from build123d import *

# Parameters (mm, degrees)
SKETCH_2_R          = 20
EXTRUDE_2_DEPTH     = 50
SKETCH_3_R          = 10
SKETCH_3_W          = 50
SKETCH_3_H          = 8
EXTRUDE_3_DEPTH     = 30
EXTRUDE_START       = -12
SKETCH_4_R          = 10
EXTRUDE_4_DEPTH     = 12
SKETCH_5_R          = 13
SKETCH_5_R_2        = 5.5
CUT_EXTRUDE_1_DEPTH = 89.593995864


with BuildPart() as part:
    # Эскиз2 → Бобышка-Вытянуть2 (new body)
    with BuildSketch(Plane.XY):
        Circle(SKETCH_2_R)
    extrude(amount=EXTRUDE_2_DEPTH)

    # Эскиз3 → Бобышка-Вытянуть3 (add)
    with BuildSketch(Plane.XY.offset(50)):
        with Locations((-50, 0)):
            Circle(SKETCH_3_R)
        with Locations((-25, 0)):
            Rectangle(SKETCH_3_W, SKETCH_3_H)
    extrude(amount=-EXTRUDE_3_DEPTH)

    # Эскиз4 → Бобышка-Вытянуть4 (add)
    with BuildSketch(Plane.XY.offset(50).offset(EXTRUDE_START)):
        with BuildLine():
            Line((-10.645829468, -16.931223079), (26.496890419, -40.285416693))
            ThreePointArc((26.496890419, -40.285416693), (24.748737342, -24.748737342), (40.285416693, -26.496890419))
            Line((40.285416693, -26.496890419), (16.931223079, 10.645829468))
            ThreePointArc((16.931223079, 10.645829468), (14.142135624, -14.142135624), (-10.645829468, -16.931223079))
        make_face()
        with Locations((31.819805153, -31.819805153)):
            Circle(SKETCH_4_R)
    extrude(amount=EXTRUDE_4_DEPTH)

    # Эскиз5 → Вырез-Вытянуть1 (cut, through all)
    with BuildSketch(Plane.XY.offset(50)):
        Circle(SKETCH_5_R)
        with Locations((-50, 0)):
            Circle(SKETCH_5_R_2)
        with Locations((31.819805153, -31.819805153)):
            Circle(SKETCH_5_R_2)
    extrude(amount=-CUT_EXTRUDE_1_DEPTH, mode=Mode.SUBTRACT)


solid = part.part
Could you check a few things on this model? Use its own coordinates, in mm. A direction names the side the tool comes from. Coordinates: 2 decimals unless noted, no trailing zeros. Write each loop counter-clockwise with the first axis right and the second up, starting at its lowest first coordinate (ties: lowest second). Pieces come first, ordered by that corner, then holes. Notation, with made-up numbers: (26.25, -28.5) - (35.25, -28.5) arc R12 ccw to (35.25, -5.5) - close; hole circle Ø2 at (33.5, -23.5). An arc over 180 degrees is marked (long way). Put each result on its own line as item: value. Start each with the question number.
Q1. I want a section at D-D on y = 0. Write out the boundary of the cut face in (x, z) (3 decimals).
Q2. I want a section at B-B on y = -28. Write out the boundary of the cut face in (x, z).
Q3. Thinking about a two-plate mould opening in X: for faces 4 (the cylindrical face through (-55.495, 0.242, 35.21)), 5 (the flat face through (28.772, -8.186, 43.916)), 6 (the cylindrical face through (-60, 0, 35)), 7 (the flat face through (-40, 0, 20)), which applies, pulls with the +X half, pulls with the -X half, needs draft (parallel to the pull), parting line crosses it, or undercut?
Q4. I want a section at C-C on z = 21.5. Write out the boundary of the cut face in (x, y).
Q5. Which directions (+Z, -Z, +X, -X, +Y, -Y) give clear straight access to the entire face, cutting with the end or side of a thin tool? Please do faces 1 (the flat face through (-30, 4, 35)), 2 (the cylindrical face through (-2.6, 19.83, 19.09)), 3 (the flat face through (-30, -4, 35)).
Q6. Please list where these lines run through material, in increasing order: L1, parallel to X at y = -6, z = 43.5; L2, parallel to Y at x = -33, z = 25; L3, parallel to X at y = -7.5, z = 28.
Q7. I'm going to push flat-ended pins straight in: P1, Ø6.5, axis at x = -32.5, z = 29.5, coming from the -Y side; P2, Ø14.5, axis at x = -50, y = 0, coming from the -Z side; P3, Ø6.5, axis at x = -30.5, z = 30.5, coming from the +Y side. Where does each tip first touch, or does it pass through?
Q8. I want a section at A-A on x = -50. Write out the boundary of the cut face in (y, z).
Checks:
1. outline: (-60, 20) - (-55.5, 20) - (-55.5, 50) - (-60, 50) - close; (-44.5, 20) - (-20, 20) - (-20, 0) - (-13, 0) - (-13, 50) - (-44.5, 50) - close; (13, 0) - (20, 0) - (20, 38) - (23.625, 38) - (23.625, 50) - (13, 50) - close
2. outline: (6.96, 38) - (27.86, 38) - (27.86, 50) - (6.96, 50) - close; (35.78, 38) - (41.06, 38) - (41.06, 50) - (35.78, 50) - close
3. face 4: undercut
3. face 5: pulls with the +X half
3. face 6: undercut
3. face 7: needs draft
4. outline: (-40.83, -4) - (-19.6, -4) arc R20 ccw (long way) to (-19.6, 4) - (-40.83, 4) arc R10 ccw (long way) to start; hole circle Ø11 at (-50, 0); hole circle Ø26 at (0, 0)
5. face 1: +Z, -Z, +Y
5. face 2: -Z
5. face 3: +Z, -Z, -Y
6. L1: -58 to -42, -19.08 to -11.53, 11.53 to 27.4
6. L2: -4 to 4
6. L3: -56.61 to -43.39, -18.54 to -10.62, 10.62 to 18.54
7. P1: y = -4
7. P2: z = 20
7. P3: y = 4
8. outline: (-10, 20) - (-5.5, 20) - (-5.5, 50) - (-10, 50) - close; (5.5, 20) - (10, 20) - (10, 50) - (5.5, 50) - close
